from build123d import *

# Parameters (mm, degrees)
SKETCH1_W           = 85.09
SKETCH1_H           = 55.88
BOSS_EXTRUDE1_DEPTH = 1.27
FILLET2_R           = 2.54
SKETCH2_R           = 1.3462
CUT_EXTRUDE1_DEPTH  = 1.27
SKETCH3_W           = 17.018
SKETCH3_H           = 13.208
BOSS_EXTRUDE2_DEPTH = 15.748
SKETCH4_W           = 21.3487
SKETCH4_H           = 15.748
BOSS_EXTRUDE3_DEPTH = 13.5128
SKETCH5_W           = 15.494
SKETCH5_H           = 11.9888
BOSS_EXTRUDE4_DEPTH = 1.651


with BuildPart() as part:
    # Sketch1 → Boss-Extrude1 (new body)
    with BuildSketch(Plane.XY):
        with Locations((42.545, 27.94)):
            Rectangle(SKETCH1_W, SKETCH1_H)
    extrude(amount=BOSS_EXTRUDE1_DEPTH)

    # Fillet2
    fillet2_edges = [part.edges().sort_by_distance(p)[0] for p in [
        (85.09, 0, 0.635),
        (0, 0, 0.635),
        (0, 55.88, 0.635),
        (85.09, 55.88, 0.635),
    ]]
    fillet(fillet2_edges, radius=FILLET2_R)

    # Sketch2 → Cut-Extrude1 (cut)
    with BuildSketch(Plane.XY.offset(1.27)):
        with Locations((81.4578, 52.2478)):
            Circle(SKETCH2_R)
        with Locations((24.7396, 52.2478)):
            Circle(SKETCH2_R)
        with Locations((24.7396, 3.6322)):
            Circle(SKETCH2_R)
        with Locations((81.4578, 3.6322)):
            Circle(SKETCH2_R)
    extrude(amount=-CUT_EXTRUDE1_DEPTH, mode=Mode.SUBTRACT)

    # Sketch3 → Boss-Extrude2 (add)
    with BuildSketch(Plane.XY.offset(1.27)):
        with Locations((6.477, 27.2288)):
            Rectangle(SKETCH3_W, SKETCH3_H)
        with Locations((6.477, 9.017)):
            Rectangle(SKETCH3_W, SKETCH3_H)
    extrude(amount=BOSS_EXTRUDE2_DEPTH)

    # Sketch4 → Boss-Extrude3 (add)
    with BuildSketch(Plane.XY.offset(1.27)):
        with Locations((8.12165, 45.6438)):
            Rectangle(SKETCH4_W, SKETCH4_H)
    extrude(amount=BOSS_EXTRUDE3_DEPTH)

    # Sketch5 → Boss-Extrude4 (add)
    with BuildSketch(Plane(origin=(0, 0, 0), x_dir=(-1, 0, 0), z_dir=(0, 0, -1))):
        with Locations((-79.2353, 27.94)):
            Rectangle(SKETCH5_W, SKETCH5_H)
    extrude(amount=BOSS_EXTRUDE4_DEPTH)


solid = part.part
Read the model definition and answer for the solid it produces. Units are mm, in the model's axes. A direction names the side the tool comes from. Round coordinates to 2 decimals unless told otherwise and drop trailing zeros. Loops run counter-clockwise (first coordinate to the right, second up) from the corner with the lowest first, then second, coordinate; pieces in that order, holes last.
Q1. Section B-B on y = 43.5 is taken. Write down the section's boundary in (x, z).
Q2. Section D-D on y = 30.5 is taken. Write down the section's boundary in (x, z), and give its area (3 significant figures).
Q3. Determine the mould class of faces 1 (the face through (23.395, 3.691, 0.644)), 2 (the face through (-2.032, 9, 9)), 3 (the face through (8, 46, 14.783)) for opening direction X: released by +X, released by -X, zero draft, split by the parting line, or undercut.
Q4. Section C-C on x = 5 is taken. Write down the section's boundary in (y, z), and give its area (3 significant figures).
Q5. Which of the six approach directions +Z, -Z, +X, -X, +Y, -Y give full straight-line access (tool end or side, diameter ignored) to faces 4 (the face through (79, 28, -1.651)), 5 (the face through (-1, 27, 1.27)), 6 (the face through (8, 37.77, 8)), 7 (the face through (14.986, 9, 9)), 8 (the face through (86, 28, 0))?
Q6. Section A-A on z = 2.5 is taken. Write down the section's boundary in (x, y).
Q7. Consider probe 1 along Y at (x, z) = (4, 16); probe 2 along X at (y, z) = (46, 12); probe 3 along Z at (x, y) = (57.5, 9.5). Determine where each line is inside the solid, lowest interval first.
Q8. Each of these flat-tipped pins is pushed along its axis until it touches: pin 1 (4.5 mm diameter, centred on x = 4.5, z = 11.5, fed in from +Y); pin 2 (4 mm diameter, centred on y = 49, z = 10.5, fed in from +X); pin 3 (8 mm diameter, centred on x = 63.5, y = 22.5, fed in from -Z). Where does it stop, or does it pass through?
Output:
1. outline: (-2.55, 1.27) - (0, 1.27) - (0, 0) - (85.09, 0) - (85.09, 1.27) - (18.8, 1.27) - (18.8, 14.78) - (-2.55, 14.78) - close
2. outline: (-2.03, 1.27) - (0, 1.27) - (0, 0) - (71.49, 0) - (71.49, -1.65) - (86.98, -1.65) - (86.98, 0) - (85.09, 0) - (85.09, 1.27) - (14.99, 1.27) - (14.99, 17.02) - (-2.03, 17.02) - close
2. area: 402 mm2
3. face 1: undercut
3. face 2: released by -X
3. face 3: zero draft
4. outline: (0, 0) - (55.88, 0) - (55.88, 1.27) - (53.52, 1.27) - (53.52, 14.78) - (37.77, 14.78) - (37.77, 1.27) - (33.83, 1.27) - (33.83, 17.02) - (20.62, 17.02) - (20.62, 1.27) - (15.62, 1.27) - (15.62, 17.02) - (2.41, 17.02) - (2.41, 1.27) - (0, 1.27) - close
4. area: 700 mm2
5. face 4: -Z, +X, -X, +Y, -Y
5. face 5: -Z, -X, +Y, -Y
5. face 6: +Z, +X, -X
5. face 7: +Z, +X, -Y
5. face 8: +Z, +X, +Y, -Y
6. outline: (-2.55, 37.77) - (18.8, 37.77) - (18.8, 53.52) - (-2.55, 53.52) - close; (-2.03, 2.41) - (14.99, 2.41) - (14.99, 15.62) - (-2.03, 15.62) - close; (-2.03, 20.62) - (14.99, 20.62) - (14.99, 33.83) - (-2.03, 33.83) - close
7. probe 1: y = 2.41 to 15.62, 20.62 to 33.83
7. probe 2: x = -2.55 to 18.8
7. probe 3: z = 0 to 1.27
8. pin 1: stops at y = 53.52
8. pin 2: stops at x = 18.8
8. pin 3: stops at z = 0
